from build123d import *

# Parameters (mm, degrees)
SKETCH_1_W                = 90
SKETCH_1_H                = 78
SKETCH_1_R                = 16
EXTRUDE_1_DEPTH           = 10
SKETCH_2_R                = 38
SKETCH_2_R_2              = 31.1
CUT_EXTRUDE_1_DEPTH       = 4
HOLE_WIZARD_1_D           = 3.2
HOLE_WIZARD_1_DEPTH       = 8.5
HOLE_WIZARD_1_CBORE_D     = 6
HOLE_WIZARD_1_CBORE_DEPTH = 3.4
HOLE_WIZARD_1_TIP         = 0.96137699
HOLE_WIZARD_4_0_4_1_D     = 4
CHAMFER_1_SIZE            = 2


with BuildPart() as part:
    # 草图1 → 凸台-拉伸1 (new body)
    with BuildSketch(Plane.XY):
        Rectangle(SKETCH_1_W, SKETCH_1_H)
        Circle(SKETCH_1_R, mode=Mode.SUBTRACT)
    extrude(amount=EXTRUDE_1_DEPTH)

    # 草图2 → 切除-拉伸1 (cut)
    with BuildSketch(Plane.XY.offset(10)):
        Circle(SKETCH_2_R)
        Circle(SKETCH_2_R_2, mode=Mode.SUBTRACT)
    extrude(amount=-CUT_EXTRUDE_1_DEPTH, mode=Mode.SUBTRACT)

    # 打孔尺寸(%根据)内六角圆柱头螺钉的类型1
    with Locations(Plane(origin=(0, 0, 0), x_dir=(-1, 0, 0), z_dir=(0, 0, -1))):
        with Locations((0, 34.5), (29.877876431, 17.25), (29.877876431, -17.25), (0, -34.5), (-29.877876431, -17.25), (-29.877876431, 17.25)):
            CounterBoreHole(HOLE_WIZARD_1_D / 2, HOLE_WIZARD_1_CBORE_D / 2, HOLE_WIZARD_1_CBORE_DEPTH, depth=HOLE_WIZARD_1_DEPTH)
            with Locations((0, 0, -(HOLE_WIZARD_1_DEPTH + HOLE_WIZARD_1_TIP / 2))):  # 118° drill point
                Cone(0, HOLE_WIZARD_1_D / 2, HOLE_WIZARD_1_TIP, mode=Mode.SUBTRACT)

    # Ø4.0 (4) 直径孔1 (through all)
    with Locations(Plane(origin=(0, 0, 0), x_dir=(-1, 0, 0), z_dir=(0, 0, -1))):
        with Locations((0, -28)):
            Hole(HOLE_WIZARD_4_0_4_1_D / 2)

    # 倒角1
    # the kernel refuses this chamfer: 2 mm, written as the material it takes off along each edge
    with BuildSketch(Plane(origin=(0, -28, 0), x_dir=(1, 0, 0), z_dir=(0, -1, 0))) as chamfer_1_piece_1:
        Polygon((2 + CHAMFER_1_SIZE, 0), (2, CHAMFER_1_SIZE), (2, 0), align=None)
    revolve(axis=Axis((0, -28, 0), (0, 0, 1)), mode=Mode.SUBTRACT)
    with BuildSketch(Plane(origin=(0, -28, 10), x_dir=(1, 0, 0), z_dir=(0, -1, 0))) as chamfer_1_piece_2:
        Polygon((2, -CHAMFER_1_SIZE), (2 + CHAMFER_1_SIZE, 0), (2, 0), align=None)
    revolve(axis=Axis((0, -28, 10), (0, 0, 1)), mode=Mode.SUBTRACT)


solid = part.part
Geometry: final body of the model. Coordinates: model frame, mm. A direction names the side the tool comes from. Give positions to 0.01 mm unless a question says otherwise; leave off trailing zeros. Order: outer loops, then holes, each group sorted by start corner. A loop starts at its lowest first (then second) coordinate and runs counter-clockwise, first axis right, second up. Notation, with made-up numbers: (78, -34.75) -> (86, -34.75) arc R15 cw to (86, -30.75) -> close; hole circle Ø4 at (13.25, 26). An arc over 180 degrees is marked (long way). Put each result on its own line as item: value.
Q1. Material intervals for L1, parallel to Y at x = 0, z = 7; L2, parallel to Y at x = 0, z = 4.3; L3, parallel to Y at x = -27, z = 8, sorted ascending.
Here are the results:
L1: y = -39 to -38, -31.1 to -30, -26 to -16, 16 to 31.1, 38 to 39
L2: y = -39 to -36.1, -32.9 to -30, -26 to -16, 16 to 32.9, 36.1 to 39
L3: y = -39 to -26.74, -15.43 to 15.43, 26.74 to 39
Q2. Section A-A, the plane y = -17.25. Return loops of the section in (x, z).
Here are the results:
outline: (-45, 0) -> (-32.88, 0) -> (-32.88, 3.4) -> (-31.48, 3.4) -> (-31.48, 6) -> (-33.86, 6) -> (-33.86, 10) -> (-45, 10) -> close; (-28.28, 3.4) -> (-26.88, 3.4) -> (-26.88, 0) -> (26.88, 0) -> (26.88, 3.4) -> (28.28, 3.4) -> (28.28, 6) -> (25.88, 6) -> (25.88, 10) -> (-25.88, 10) -> (-25.88, 6) -> (-28.28, 6) -> close; (31.48, 3.4) -> (32.88, 3.4) -> (32.88, 0) -> (45, 0) -> (45, 10) -> (33.86, 10) -> (33.86, 6) -> (31.48, 6) -> close
Q3. Reachability of faces 1 (the face through (-31.06, -16.17, 4.72)), 2 (the face through (17.535, -33.713, 8.028)), 3 (the face through (32.259, -19.075, 1.676)) from +Z, -Z, +X, -X, +Y, -Y: full face, straight path, thin tool, end or side. Return the list, or none.
Here are the results:
face 1: +Z, -Z
face 2: +Z
face 3: -Z
Q4. Section B-B, the plane x = 14. Return loops of the section in (y, z).
Here are the results:
outline: (-39, 0) -> (-7.75, 0) -> (-7.75, 10) -> (-27.77, 10) -> (-27.77, 6) -> (-35.33, 6) -> (-35.33, 10) -> (-39, 10) -> close; (7.75, 0) -> (39, 0) -> (39, 10) -> (35.33, 10) -> (35.33, 6) -> (27.77, 6) -> (27.77, 10) -> (7.75, 10) -> close
Q5. Pin query (flat end, axial travel): pin 1 (23 mm diameter, centred on x = -9, y = -9, fed in from +Z); pin 2 (3 mm diameter, centred on x = 0, y = 34.5, fed in from -Z); pin 3 (1.8 mm diameter, centred on x = -29, y = -17.5, fed in from -Z); pin 4 (5 mm diameter, centred on x = -29.88, y = 17.25, fed in from +Z). Return the tip coordinate at first contact, or that it passes through.
Here are the results:
pin 1: stops at z = 10
pin 2: passes through
pin 3: stops at z = 3.4
pin 4: stops at z = 6
Q6. Section D-D, the plane y = 26. Return loops of the section in (x, z), then the cut area to 3 significant figures.
Here are the results:
outline: (-45, 0) -> (45, 0) -> (45, 10) -> (27.71, 10) -> (27.71, 6) -> (17.06, 6) -> (17.06, 10) -> (-17.06, 10) -> (-17.06, 6) -> (-27.71, 6) -> (-27.71, 10) -> (-45, 10) -> close
area: 815 mm^2
Q7. Section C-C, the plane y = -28. Return loops of the section in (x, z).
Here are the results:
outline: (-45, 0) -> (-4, 0) -> (-2, 2) -> (-2, 8) -> (-4, 10) -> (-13.54, 10) -> (-13.54, 6) -> (-25.69, 6) -> (-25.69, 10) -> (-45, 10) -> close; (2, 2) -> (4, 0) -> (45, 0) -> (45, 10) -> (25.69, 10) -> (25.69, 6) -> (13.54, 6) -> (13.54, 10) -> (4, 10) -> (2, 8) -> close
